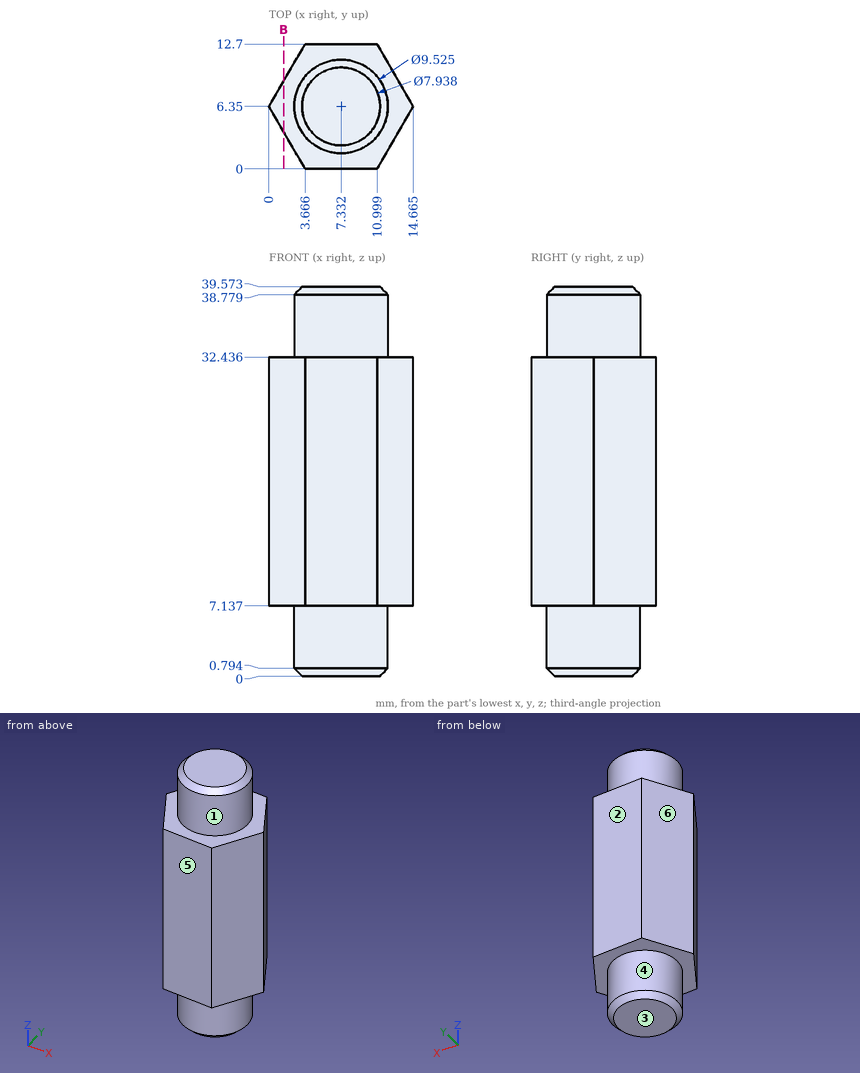
Input: dimensioned drawing with shaded views. Units: mm. Origin: part minimum x, y, z. A direction names the side the tool comes from. Round coordinates to 2 decimals unless told otherwise and drop trailing zeros. Order: outer loops, then holes, each group sorted by start corner. A loop starts at its lowest first (then second) coordinate and runs counter-clockwise, first axis right, second up.
Q1. Section B-B, the plane x = 1.5. Output: boundary loops of the cut face in (y, z) (1 decimal).
Result sheet:
outline: (3.8, 7.1) - (8.9, 7.1) - (8.9, 32.4) - (3.8, 32.4) - close
Q2. Access query for the marked faces 1 and 2. Directions: +Z, -Z, +X, -X, +Y, -Y. A direction counts if a zero-diameter tool reaches every point of the face in a straight line with its end or side. Return the directions, or none.
Result sheet:
face 1: +Z
face 2: +Z, -Z, +X, -X, +Y
Q3. Material intervals for probe 1 along Z at (x, y) = (12.5, 6) (1 decimal); probe 2 along Y at (x, z) = (12.25, 23) (1 decimal); probe 3 along Y at (x, z) = (4.5, 33.5), sorted ascending.
Result sheet:
probe 1: z = 7.1 to 32.4
probe 2: y = 2.2 to 10.5
probe 3: y = 2.52 to 10.18
Q4. Mould query, pull axis Y, two halves, no side actions, for the marked faces 3, 4, 5 and 6. Classes: released by +Y, released by -Y, zero draft, split by the parting line, or undercut.
Result sheet:
face 3: zero draft
face 4: split by the parting line
face 5: released by -Y
face 6: released by +Y
Q5. Pin query (flat end, axial travel): pin 1 (5 mm diameter, centred on y = 2.5, z = 14, fed in from -X); pin 2 (1 mm diameter, centred on y = 2, z = 18, fed in from +X); pin 3 (6 mm diameter, centred on x = 8.5, z = 18, fed in from -Y); pin 4 (1 mm diameter, centred on y = 8, z = 18.5, fed in from -X) (1 decimal). Return the tip coordinate at first contact, or that it passes through.
Result sheet:
pin 1: stops at x = 0.78
pin 2: stops at x = 12.44
pin 3: stops at y = 0
pin 4: stops at x = 0.7
